Source: CAD feature listing. Evaluate the final solid. Frame: model axes, mm. Face numbers are marked on the shaded views. A direction names the side the tool comes from. Round coordinates to 2 decimals unless told otherwise and drop trailing zeros. Loops run counter-clockwise (first coordinate to the right, second up) from the corner with the lowest first, then second, coordinate; pieces in that order, holes last. Notation, with made-up numbers: (89.5, 88) -> (124.5, 88) arc R21 cw to (124.5, 122) -> close; hole circle Ø8 at (22.25, -21). An arc over 180 degrees is marked (long way). Put each result on its own line as item: value. Start each with the question number.
1. Draft query along Y for the marked faces 1, 2 and 3. Return one class per face: pulls with the +Y half, pulls with the -Y half, needs draft (parallel to the pull), parting line crosses it, or undercut.
2. Cut plane A-A (y = -13). Return the cut outline in (x, z), then the cut area to 3 significant figures.
3. Material intervals for L1, parallel to Z at x = 5.25, y = -8.5; L2, parallel to Z at x = 1.5, y = -7; L3, parallel to Z at x = 13.5, y = 14.5, sorted ascending.
4. Cut plane D-D (y = 3). Return the cut outline in (x, z).
5. Cut plane C-C (z = 9). Return the cut outline in (x, y).
6. Set-up query: the marked faces 4 and 5. Return all of +Z, -Z, +X, -X, +Y, -Y with unobstructed straight access to the full face (end or side cutting, diameter ignored); none if empty.
7. Contact query for flat-ended pins moving along their axis: pin 1 (2 mm diameter, centred on x = 9.5, y = 11, fed in from -Z); pin 2 (6 mm diameter, centred on y = -8.83, z = 8.83, fed in from -X); pin 3 (6 mm diameter, centred on x = 6, z = -7.5, fed in from +Y); pin 4 (12 mm diameter, centred on y = -15.5, z = 5.5, fed in from -X). Output: stop coordinate, or through.
8. Cut plane B-B (x = 12.5). Return the cut outline in (y, z).
```python
from build123d import *

# Parameters (mm, degrees)
SKIZZE1_R                       = 5
AUFSATZ_LINEAR_AUSTRAGEN1_DEPTH = 20


with BuildPart() as part:
    # Skizze1 → Aufsatz-Linear austragen1 (new body)
    with BuildSketch(Plane(origin=(0, 0, 0), x_dir=(0, 0, -1), z_dir=(1, 0, 0))):
        Polygon((0, 0), (0, 20), (-10.600988733, 20), (-25.787709792, 4.813278942), (-25.787709792, -25.787709792), (4.813278942, -25.787709792), (20, -10.600988733), (20, 0), align=None)
        with Locations((-8.83007243, -8.83007243)):
            Circle(SKIZZE1_R, mode=Mode.SUBTRACT)
    extrude(amount=AUFSATZ_LINEAR_AUSTRAGEN1_DEPTH)


solid = part.part
```
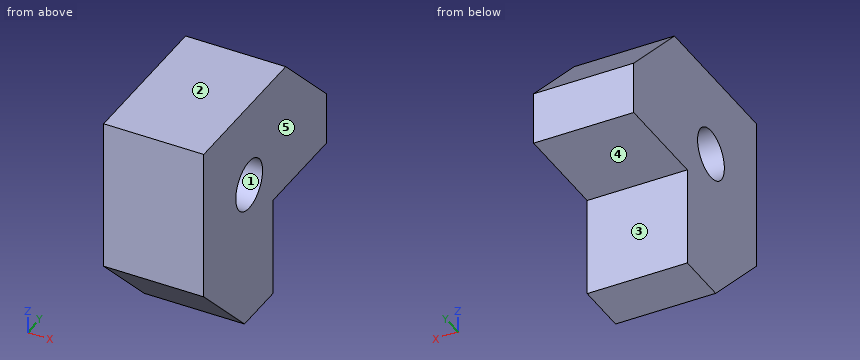
Solution:
1. face 1: undercut
1. face 2: needs draft
1. face 3: pulls with the +Y half
2. outline: (0, -17.6) -> (20, -17.6) -> (20, 6.07) -> (0, 6.07) -> close; (0, 11.59) -> (20, 11.59) -> (20, 25.79) -> (0, 25.79) -> close
2. area: 757 mm^2
3. L1: z = -20 to 3.84, 13.82 to 25.79
3. L2: z = -20 to 4.18, 13.48 to 25.79
3. L3: z = 0 to 16.1
4. outline: (0, 0) -> (20, 0) -> (20, 25.79) -> (0, 25.79) -> close
5. outline: (0, -25.79) -> (20, -25.79) -> (20, -13.83) -> (0, -13.83) -> close; (0, -3.83) -> (20, -3.83) -> (20, 20) -> (0, 20) -> close
6. face 4: -Z, +X, -X, +Y
6. face 5: +Z, -Z, +X, +Y, -Y
7. pin 1: stops at z = 0
7. pin 2: passes through
7. pin 3: stops at y = 0
7. pin 4: stops at x = 0
8. outline: (-25.79, -4.81) -> (-10.6, -20) -> (0, -20) -> (0, 0) -> (20, 0) -> (20, 10.6) -> (4.81, 25.79) -> (-25.79, 25.79) -> close; hole circle Ø10 at (-8.83, 8.83)
